Work out the finished part from the listing and answer in its coordinate system (mm). Face numbers are marked on the shaded views. A direction names the side the tool comes from. Round coordinates to 2 decimals unless told otherwise and drop trailing zeros. Order: outer loops, then holes, each group sorted by start corner. A loop starts at its lowest first (then second) coordinate and runs counter-clockwise, first axis right, second up. Notation, with made-up numbers: M -26.75,43.5 L -21.75,43.5 A26 ccw -21.75,59.5 Z; hole C 11,29.25 d3. An arc over 180 degrees is marked long. Return JSON: item names as keys, results as strings.
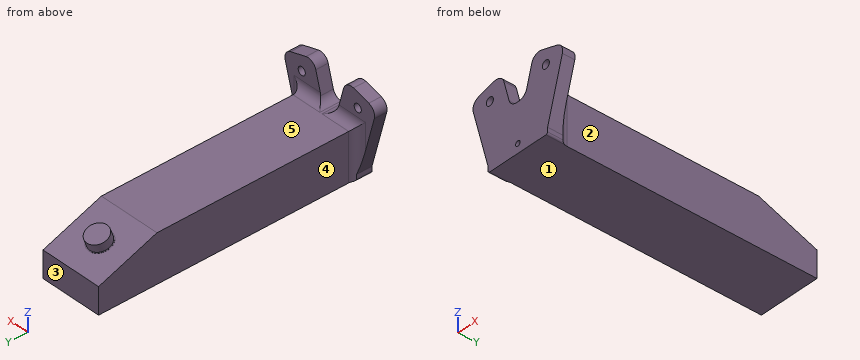
from build123d import *

# Parameters (mm, degrees)
AUFSATZ_LINEAR_AUSTRAGEN1_DEPTH = 35
SKIZZE3_R                       = 6
AUFSATZ_LINEAR_AUSTRAGEN2_DEPTH = 5
SKIZZE4_R                       = 6.5
AUFSATZ_LINEAR_AUSTRAGEN3_DEPTH = 0.1
SKIZZE9_R                       = 1.425
SCHNITT_LINEAR_AUSTRAGEN2_DEPTH = 10
SKIZZE10_R                      = 2.25
AUFSATZ_LINEAR_AUSTRAGEN4_DEPTH = 7
VERRUNDUNG1_R                   = 5
VERRUNDUNG2_R                   = 1


with BuildPart() as part:
    # Skizze1 → Aufsatz-Linear austragen1 (new body)
    with BuildSketch(Plane(origin=(0, 0, 0), x_dir=(0, 0, -1), z_dir=(1, 0, 0))):
        Polygon((0, 0), (11.970705016, 0), (26.82, 0), (26.82, 152.889241728), (11.970705016, 152.889241728), (0, 120), align=None)
    extrude(amount=AUFSATZ_LINEAR_AUSTRAGEN1_DEPTH)

    # Skizze3 → Aufsatz-Linear austragen2 (add)
    with BuildSketch(Plane(origin=(0, 14.037333413, 38.567256581), x_dir=(1, 0, 0), z_dir=(0, 0.342020143, 0.939692621))):
        with Locations((17.5, 130.263114494)):
            Circle(SKIZZE3_R)
    extrude(amount=AUFSATZ_LINEAR_AUSTRAGEN2_DEPTH)

    # Skizze4 → Aufsatz-Linear austragen3 (add)
    with BuildSketch(Plane(origin=(0, 14.037333413, 38.567256581), x_dir=(1, 0, 0), z_dir=(0, 0.342020143, 0.939692621))):
        with Locations((17.5, 130.263114494)):
            Circle(SKIZZE4_R)
    extrude(amount=AUFSATZ_LINEAR_AUSTRAGEN3_DEPTH)

    # Skizze9 → Schnitt-Linear austragen2 (cut)
    with BuildSketch(Plane.XZ):
        with Locations((17.498844944, -21.644236877)):
            Circle(SKIZZE9_R)
    extrude(amount=-SCHNITT_LINEAR_AUSTRAGEN2_DEPTH, mode=Mode.SUBTRACT)

    # Skizze10 → Aufsatz-Linear austragen4 (add)
    with BuildSketch(Plane.XZ):
        Polygon((35, -26.82), (36.222689888, -26.82), (36.222689888, -23.396698607), (46.889907729, 14.777378017), (27.627810102, 20.159904842), (21.994403466, 0), align=None)
        with Locations((35.124354886, 9.830031101)):
            Circle(SKIZZE10_R, mode=Mode.SUBTRACT)
        Polygon((-1.222689888, -26.82), (-1.222689888, -23.396698607), (-11.889907729, 14.777378017), (7.372189898, 20.159904842), (13.005596534, 0), (0, -26.82), align=None)
        with Locations((-0.124354886, 9.830031101)):
            Circle(SKIZZE10_R, mode=Mode.SUBTRACT)
    extrude(amount=-AUFSATZ_LINEAR_AUSTRAGEN4_DEPTH)

    # Verrundung1
    verrundung1_edges = [part.edges().sort_by_distance(p)[0] for p in [
        (6.502798267, 7, 0),
        (28.497201733, 7, 0),
        (35, 7, -13.41),
        (0, 7, -13.41),
        (-11.889907729, 3.5, 14.777378017),
        (7.372189898, 3.5, 20.159904842),
        (46.889907729, 3.5, 14.777378017),
        (27.627810102, 3.5, 20.159904842),
        (21.994403466, 3.5, 0),
        (13.005596534, 3.5, 0),
    ]]
    fillet(verrundung1_edges, radius=VERRUNDUNG1_R)

    # Verrundung2
    verrundung2_edges = [part.edges().sort_by_distance(p)[0] for p in [
        (36.222689888, 4.362018901, -26.82),
        (-1.222689888, 4.362018901, -26.82),
    ]]
    fillet(verrundung2_edges, radius=VERRUNDUNG2_R)


solid = part.part
Item 1: Find section A-A (y = 30.5). Determine the outline of the cut face in (x, z).
Output:
{"outline": "M 0,-26.82 L 35,-26.82 L 35,0 L 0,0 Z"}
Item 2: Each of these flat-tipped pins is pushed along its axis until it touches: pin 1 (5 mm diameter, centred on x = 34.5, y = 55.5, fed in from +Z); pin 2 (11 mm diameter, centred on x = 29.5, z = 6, fed in from +Y); pin 3 (4 mm diameter, centred on y = 82, z = -7, fed in from +X); pin 4 (3.5 mm diameter, centred on x = 17.5, z = -21.64, fed in from -Y). Where does it stop, or does it pass through?
Output:
{"pin 1": "stops at z = 0", "pin 2": "stops at y = 9.82", "pin 3": "stops at x = 35", "pin 4": "stops at y = 0"}
Item 3: Find section B-B (z = -16.5). Determine the outline of the cut face in (x, y).
Output:
{"outline": "M -3.15,0 L 38.15,0 L 38.15,7.35 A5 cw 35,12 L 35,152.89 L 0,152.89 L 0,12 A5 cw -3.15,7.35 Z"}
Item 4: Find section C-C (x = 31). Determine the outline of the cut face in (y, z).
Output:
{"outline": "M 0,-26.82 L 152.89,-26.82 L 152.89,-11.97 L 120,0 L 12,0 A5 cw 7,5 L 7,19 L 0,19 Z"}
Item 5: The mould has two halves that part along Y. Classify the marked faces 3, 4 and 5: pulls with the +Y half, pulls with the -Y half, needs draft (parallel to the pull), parting line crosses it, or undercut.
Output:
{"face 3": "pulls with the +Y half", "face 4": "needs draft", "face 5": "undercut"}
Item 6: Which of the six approach directions +Z, -Z, +X, -X, +Y, -Y give full straight-line access (tool end or side, diameter ignored) to the marked faces 1 and 2?
Output:
{"face 1": "-Z, +X, -X, +Y, -Y", "face 2": "+Z, -Z, +X, +Y"}
Item 7: Consider line 1 along X through (y, z) = (121, -8.5); line 2 along Z through (x, y) = (20.5, 39); line 3 along Y through (x, z) = (2, 8). Determine where each line is inside the solid, lowest interval first. Write a range as [from, to].
Output:
{"line 1": "x = [0, 35]", "line 2": "z = [-26.82, 0]", "line 3": "y = [0, 7]"}
